Study the drawing (mm; zero at the part's minimum x, y, z) and answer. A direction names the side the tool comes from. Give positions to 0.01 mm unless a question says otherwise; leave off trailing zeros. Order: outer loops, then holes, each group sorted by start corner. A loop starts at its lowest first (then second) coordinate and runs counter-clockwise, first axis right, second up. Notation, with made-up numbers: (20.5, -36.75) - (59.5, -36.75) arc R24 cw to (59.5, -9.75) - close; hole circle Ø10 at (-36.5, 25.5). An arc over 180 degrees is marked (long way). Return JSON: item names as keys, results as strings.
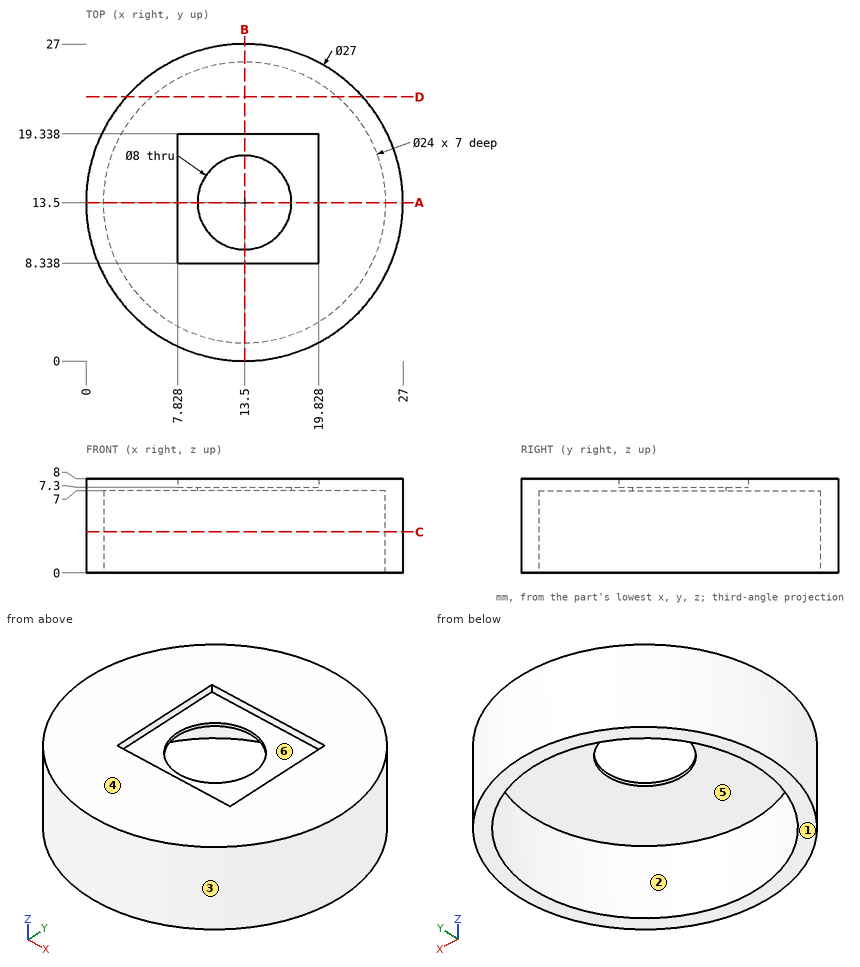
Q1. Consider L1, parallel to Y at x = 13.5, z = 5; L2, parallel to Y at x = 13.5, z = 7.25; L3, parallel to Z at x = 17, y = 4.5. Determine where each line is inside the solid, lowest interval first.
Values:
{"L1": "y = 0 to 1.5, 25.5 to 27", "L2": "y = 0 to 9.5, 17.5 to 27", "L3": "z = 7 to 8"}
Q2. For the marked faces 1 and 2, determine the directions among +Z, -Z, +X, -X, +Y, -Y from which every point of the face is accessible in a straight line to the end or side of a thin tool.
Values:
{"face 1": "-Z, +X, -X, +Y, -Y", "face 2": "-Z"}
Q3. Given pin 1 (2 mm diameter, centred on x = 4.5, z = 6, fed in from -Y) (1 decimal); pin 2 (1.5 mm diameter, centred on y = 24, z = 4.5, fed in from +X); pin 3 (0.8 mm diameter, centred on x = 15, z = 7.5, fed in from +Y) (1 decimal), each flat-ended and moving along its own axis, determine where each tip first touches the part or whether it passes through.
Values:
{"pin 1": "stops at y = 2.6", "pin 2": "stops at x = 22.84", "pin 3": "stops at y = 27"}
Q4. A cutting plane is placed at D-D (y = 22.5). Write down the section's boundary in (x, z).
Values:
{"outline": "(3.44, 0) - (5.56, 0) - (5.56, 7) - (21.44, 7) - (21.44, 0) - (23.56, 0) - (23.56, 8) - (3.44, 8) - close"}
Q5. A cutting plane is placed at C-C (z = 3.5). Write down the section's boundary in (x, y).
Values:
{"outline": "circle Ø27 at (13.5, 13.5); hole circle Ø24 at (13.5, 13.5)"}
Q6. Determine the mould class of the marked faces 3, 4, 5 and 6 for opening direction X: released by +X, released by -X, zero draft, split by the parting line, or undercut.
Values:
{"face 3": "split by the parting line", "face 4": "zero draft", "face 5": "undercut", "face 6": "undercut"}
Q7. A cutting plane is placed at B-B (x = 13.5). Write down the section's boundary in (y, z), and give its area (3 significant figures).
Values:
{"outline": "(0, 0) - (1.5, 0) - (1.5, 7) - (9.5, 7) - (9.5, 7.3) - (8.34, 7.3) - (8.34, 8) - (0, 8) - close; (17.5, 7) - (25.5, 7) - (25.5, 0) - (27, 0) - (27, 8) - (19.34, 8) - (19.34, 7.3) - (17.5, 7.3) - close", "area": "37.9 mm²"}
Q8. A cutting plane is placed at A-A (y = 13.5). Write down the section's boundary in (x, z).
Values:
{"outline": "(0, 0) - (1.5, 0) - (1.5, 7) - (9.5, 7) - (9.5, 7.3) - (7.83, 7.3) - (7.83, 8) - (0, 8) - close; (17.5, 7) - (25.5, 7) - (25.5, 0) - (27, 0) - (27, 8) - (19.83, 8) - (19.83, 7.3) - (17.5, 7.3) - close"}
